CAD build for the part. Positions are in the model's coordinates, mm. A direction names the side the tool comes from. Give positions to 0.01 mm unless a question says otherwise; leave off trailing zeros. Order: outer loops, then holes, each group sorted by start corner. A loop starts at its lowest first (then second) coordinate and runs counter-clockwise, first axis right, second up.
from build123d import *

# Parameters (mm, degrees)
BOSS_EXTRU_5_DEPTH = 3


with BuildPart() as part:
    # Esquisse5 → Boss.-Extru.5 (new body)
    with BuildSketch(Plane.XY):
        with BuildLine():
            Line((-17.14036809, 14.446568203), (-17.14036809, 17.446568203))
            Line((-17.14036809, 17.446568203), (-9.14036809, 17.446568203))
            Line((-9.14036809, 17.446568203), (-9.14036809, -6.553431797))
            Line((-9.14036809, -6.553431797), (-14.14036809, -6.553431797))
            Line((-14.14036809, -6.553431797), (-14.14036809, -3.553431797))
            Line((-14.14036809, -3.553431797), (-45.64036809, -3.553431797))
            Line((-45.64036809, -3.553431797), (-45.64036809, 0.446568203))
            Line((-45.64036809, 0.446568203), (-44.14036809, 0.446568203))
            Line((-44.14036809, 0.446568203), (-44.14036809, 3.446568203))
            Line((-44.14036809, 3.446568203), (-45.64036809, 3.446568203))
            Line((-45.64036809, 3.446568203), (-45.64036809, 7.446568203))
            Line((-45.64036809, 7.446568203), (-48.64036809, 7.446568203))
            Line((-48.64036809, 7.446568203), (-48.64036809, 3.446568203))
            Line((-48.64036809, 3.446568203), (-50.14036809, 3.446568203))
            Line((-50.14036809, 3.446568203), (-50.14036809, 0.446568203))
            Line((-50.14036809, 0.446568203), (-48.64036809, 0.446568203))
            Line((-48.64036809, 0.446568203), (-48.64036809, -3.553431797))
            Line((-48.64036809, -3.553431797), (-61.14036809, -3.553431797))
            Line((-61.14036809, -3.553431797), (-61.14036809, -6.553431797))
            Line((-61.14036809, -6.553431797), (-69.14036809, -6.553431797))
            Line((-69.14036809, -6.553431797), (-69.14036809, 10.446568203))
            Line((-69.14036809, 10.446568203), (-60.14036809, 10.446568203))
            ThreePointArc((-60.14036809, 10.446568203), (-57.311940966, 11.618141078), (-56.14036809, 14.446568203))
            Line((-56.14036809, 14.446568203), (-56.14036809, 17.446568203))
            Line((-56.14036809, 17.446568203), (-47.14036809, 17.446568203))
            Line((-47.14036809, 17.446568203), (-47.14036809, 14.446568203))
            Line((-47.14036809, 14.446568203), (-32.64036809, 14.446568203))
            Line((-32.64036809, 14.446568203), (-32.64036809, 10.446568203))
            Line((-32.64036809, 10.446568203), (-34.14036809, 10.446568203))
            Line((-34.14036809, 10.446568203), (-34.14036809, 7.446568203))
            Line((-34.14036809, 7.446568203), (-32.64036809, 7.446568203))
            Line((-32.64036809, 7.446568203), (-32.64036809, 3.446568203))
            Line((-32.64036809, 3.446568203), (-29.64036809, 3.446568203))
            Line((-29.64036809, 3.446568203), (-29.64036809, 7.446568203))
            Line((-29.64036809, 7.446568203), (-28.14036809, 7.446568203))
            Line((-28.14036809, 7.446568203), (-28.14036809, 10.446568203))
            Line((-28.14036809, 10.446568203), (-29.64036809, 10.446568203))
            Line((-29.64036809, 10.446568203), (-29.64036809, 14.446568203))
            Line((-29.64036809, 14.446568203), (-17.14036809, 14.446568203))
        make_face()
    extrude(amount=BOSS_EXTRU_5_DEPTH)


solid = part.part
1. Pin check, flat tips, straight feed: P1, Ø0.9, axis at x = -47.5, z = 1.5, coming from the -Y side; P2, Ø1.2, axis at x = -44.5, z = 1, coming from the -Y side. Stop position of each tip, or through.
2. Saw through at A-A on y = 15.75. Give the cut face in (x, z).
3. Saw through at C-C on y = 8.25. Give the cut face in (x, z), plus the area to 3 significant figures.
4. 3-axis set-ups, long thin cutter, end or side, ignore diameter. For faces 1 (the flat face through (-52, 17.447, 1)), 2 (the flat face through (-17.14, 16, 1)), 3 (the flat face through (-45.64, -2, 1)): which of +Z, -Z, +X, -X, +Y, -Y reach the whole face in a straight line?
5. Wall check: line 1 (X direction, y = 5, z = 1.3); line 2 (X direction, y = 2, z = 1.95); line 3 (X direction, y = -4.5, z = 1.15). Give the ranges that are in metal, low to high.
6. Mould opens along Y. For faces 4 (the flat face through (-65, 10.447, 1)), 5 (the flat face through (-29, 7.447, 1)), 6 (the flat face through (-9.14, 6, 1)), 7 (the flat face through (-50.14, 2, 1)) say: released by +Y, released by -Y, zero draft, split by the parting line, or undercut.
7. Saw through at B-B on y = 4.75. Give the cut face in (x, z).
8. Saw through at D-D on x = -19.5. Give the cut face in (y, z), plus the area to 3 significant figures.
Reported:
1. P1: stops at y = 7.45
1. P2: stops at y = -3.55
2. outline: (-56.14, 0) - (-47.14, 0) - (-47.14, 3) - (-56.14, 3) - close; (-17.14, 0) - (-9.14, 0) - (-9.14, 3) - (-17.14, 3) - close
3. outline: (-69.14, 0) - (-34.14, 0) - (-34.14, 3) - (-69.14, 3) - close; (-28.14, 0) - (-9.14, 0) - (-9.14, 3) - (-28.14, 3) - close
3. area: 162 mm2
4. face 1: +Z, -Z, +X, -X, +Y
4. face 2: +Z, -Z, +Y
4. face 3: +Z, -Z, -Y
5. line 1: x = -69.14 to -48.64, -45.64 to -32.64, -29.64 to -9.14
5. line 2: x = -69.14 to -50.14, -44.14 to -9.14
5. line 3: x = -69.14 to -61.14, -14.14 to -9.14
6. face 4: released by +Y
6. face 5: undercut
6. face 6: zero draft
6. face 7: undercut
7. outline: (-69.14, 0) - (-48.64, 0) - (-48.64, 3) - (-69.14, 3) - close; (-45.64, 0) - (-32.64, 0) - (-32.64, 3) - (-45.64, 3) - close; (-29.64, 0) - (-9.14, 0) - (-9.14, 3) - (-29.64, 3) - close
8. outline: (-3.55, 0) - (14.45, 0) - (14.45, 3) - (-3.55, 3) - close
8. area: 54.0 mm2
